```python
from build123d import *

# Parameters (mm, degrees)
SKETCH1_W           = 43
SKETCH1_H           = 68.5
BOSS_EXTRUDE1_DEPTH = 5
SKETCH2_W           = 16
SKETCH2_H           = 68.5
BOSS_EXTRUDE2_DEPTH = 5
CUT_EXTRUDE1_REACH  = 62.855
SKETCH3_R           = 2.35
FILLET1_R           = 1
CHAMFER1_SIZE       = 1


with BuildPart() as part:
    # Sketch1 → Boss-Extrude1 (new body)
    with BuildSketch(Plane(origin=(0, 0, 0), x_dir=(1, 0, 0), z_dir=(0, 1, 0))):
        with Locations((8.893910561, -17.51450999)):
            Rectangle(SKETCH1_W, SKETCH1_H)
    extrude(amount=BOSS_EXTRUDE1_DEPTH)

    # Sketch2 → Boss-Extrude2 (add)
    with BuildSketch(Plane(origin=(0, 5, 0), x_dir=(1, 0, 0), z_dir=(0, 1, 0))):
        with Locations((-15.606089439, -17.51450999)):
            Rectangle(SKETCH2_W, SKETCH2_H)
    boss_extrude2 = extrude(amount=BOSS_EXTRUDE2_DEPTH)

    # Sketch3 → Cut-Extrude1 (cut, up to next)
    with BuildSketch(Plane(origin=(0, 10, 0), x_dir=(1, 0, 0), z_dir=(0, 1, 0)), mode=Mode.PRIVATE) as cut_extrude1_sk1:
        with Locations(Location((-18.106089439, 8.23549001, 0), (0, 0, 270))):
            Circle(SKETCH3_R)
    cut_extrude1_tool1 = extrude(cut_extrude1_sk1.sketch, amount=-CUT_EXTRUDE1_REACH, mode=Mode.PRIVATE) & part.part
    # Sketch3 → Cut-Extrude1 (cut, up to next)
    with BuildSketch(Plane(origin=(0, 10, 0), x_dir=(1, 0, 0), z_dir=(0, 1, 0)), mode=Mode.PRIVATE) as cut_extrude1_sk2:
        with Locations(Location((-18.106089439, -8.931176657, 0), (0, 0, 270))):
            Circle(SKETCH3_R)
    cut_extrude1_tool2 = extrude(cut_extrude1_sk2.sketch, amount=-CUT_EXTRUDE1_REACH, mode=Mode.PRIVATE) & part.part
    # Sketch3 → Cut-Extrude1 (cut, up to next)
    with BuildSketch(Plane(origin=(0, 10, 0), x_dir=(1, 0, 0), z_dir=(0, 1, 0)), mode=Mode.PRIVATE) as cut_extrude1_sk3:
        with Locations(Location((-18.106089439, -26.097843324, 0), (0, 0, 270))):
            Circle(SKETCH3_R)
    cut_extrude1_tool3 = extrude(cut_extrude1_sk3.sketch, amount=-CUT_EXTRUDE1_REACH, mode=Mode.PRIVATE) & part.part
    # Sketch3 → Cut-Extrude1 (cut, up to next)
    with BuildSketch(Plane(origin=(0, 10, 0), x_dir=(1, 0, 0), z_dir=(0, 1, 0)), mode=Mode.PRIVATE) as cut_extrude1_sk4:
        with Locations(Location((-18.106089439, -43.26450999, 0), (0, 0, 270))):
            Circle(SKETCH3_R)
    cut_extrude1_tool4 = extrude(cut_extrude1_sk4.sketch, amount=-CUT_EXTRUDE1_REACH, mode=Mode.PRIVATE) & part.part
    cut_extrude1_1 = cut_extrude1_tool1.solids().sort_by_distance((-18.106089, 10, -8.23549))[0]
    add(cut_extrude1_1, mode=Mode.SUBTRACT)
    cut_extrude1_2 = cut_extrude1_tool2.solids().sort_by_distance((-18.106089, 10, 8.931177))[0]
    add(cut_extrude1_2, mode=Mode.SUBTRACT)
    cut_extrude1_3 = cut_extrude1_tool3.solids().sort_by_distance((-18.106089, 10, 26.097843))[0]
    add(cut_extrude1_3, mode=Mode.SUBTRACT)
    cut_extrude1_4 = cut_extrude1_tool4.solids().sort_by_distance((-18.106089, 10, 43.26451))[0]
    add(cut_extrude1_4, mode=Mode.SUBTRACT)
    cut_extrude1 = cut_extrude1_1 + cut_extrude1_2 + cut_extrude1_3 + cut_extrude1_4  # Cut-Extrude1 as one shape, for the pattern or mirror that repeats it

    # Mirror1: Boss-Extrude2, Cut-Extrude1 across plane
    add(boss_extrude2.mirror(Plane(origin=(8.893910561, 0, 0), x_dir=(0, 0, 1), z_dir=(1, 0, 0))))
    add(cut_extrude1.mirror(Plane(origin=(8.893910561, 0, 0), x_dir=(0, 0, 1), z_dir=(1, 0, 0))), mode=Mode.SUBTRACT)

    # Fillet1
    fillet1_edges = [part.edges().sort_by_distance(p)[0] for p in [
        (30.393910561, 5, 17.51450999),
        (-7.606089439, 5, 17.51450999),
        (-23.606089439, 5, 17.51450999),
        (-7.606089439, 10, 17.51450999),
        (41.393910561, 5, 17.51450999),
        (25.393910561, 10, 17.51450999),
        (-12.606089439, 5, 17.51450999),
        (25.393910561, 5, 17.51450999),
    ]]
    fillet(fillet1_edges, radius=FILLET1_R)

    # Chamfer1
    chamfer1_edges = [part.edges().sort_by_distance(p)[0] for p in [
        (-18.106089439, 5, -10.58549001),
        (-18.106089439, 5, 6.581176657),
        (-18.106089439, 5, 23.747843324),
        (-18.106089439, 5, 40.91450999),
        (35.893910561, 5, -10.58549001),
        (35.893910561, 5, 6.581176657),
        (35.893910561, 5, 23.747843324),
        (35.893910561, 5, 40.91450999),
    ]]
    chamfer(chamfer1_edges, length=CHAMFER1_SIZE)


solid = part.part
```
Here's how the part is built. I have some questions about the finished solid (model axes, mm). A direction names the side the tool comes from. Give positions to 0.01 mm unless a question says otherwise; leave off trailing zeros. Write each loop counter-clockwise with the first axis right and the second up, starting at its lowest first coordinate (ties: lowest second). Pieces come first, ordered by that corner, then holes.
(1) Imagine slicing it at A-A, the plane y = 7. Count the separate pieces of the cut face and the enclosed holes in it, and give its area (3 significant figures).
Output values:
separate pieces: 2
enclosed holes: 8
area: 2,050 mm2
(2) On a 3-axis mill with a long thin cutter (end or side, diameter ignored), from which of +Z, -Z, +X, -X, +Y, -Y can I reach the whole of each face in a straight line? I mean faces 4 (the face through (-18, 5, 17)), 5 (the face through (9, 5, 17)), 6 (the face through (36, 5, 17)). Say none if no direction works.
Output values:
face 4: +Z, -Z, -X, -Y
face 5: +Z, -Z, +Y
face 6: +Z, -Z, +X, -Y
(3) Imagine slicing it at D-D, the plane y = 1. Write out the boundary of the cut face in (x, z).
Output values:
outline: (-12.61, -16.74) - (30.39, -16.74) - (30.39, 51.76) - (-12.61, 51.76) - close
(4) If I drill on L1, parallel to X at y = 8.5, z = -11.5; L2, parallel to Z at x = -19.5, y = 8.25; L3, parallel to X at y = 5.5, z = 8.5, over which ranges is the centre line in solid material (lowest first)?
Output values:
L1: x = -23.61 to -7.61, 25.39 to 41.39
L2: z = -16.74 to -10.13, -6.34 to 7.04, 10.82 to 24.21, 27.99 to 41.37, 45.16 to 51.76
L3: x = -23.47 to -20.92, -15.29 to -7.47, 25.26 to 33.08, 38.71 to 41.26
(5) Imagine slicing it at C-C, the plane x = 8.5. Write out the boundary of the cut face in (y, z), and give its area (4 significant figures).
Output values:
outline: (0, -16.74) - (5, -16.74) - (5, 51.76) - (0, 51.76) - close
area: 342.5 mm2
(6) Thinking about a two-plate mould opening in Z: for faces 1 (the face through (34.306, 8.028, 24.366)), 2 (the face through (9, 4, -16.735)), 3 (the face through (-7.606, 7, 18)), which applies, pulls with the +Z half, pulls with the -Z half, needs draft (parallel to the pull), parting line crosses it, or undercut?
Output values:
face 1: undercut
face 2: pulls with the -Z half
face 3: needs draft
(7) Will these pins go through, and if not, where does the flat tip stop? pin 1 (4 mm diameter, centred on x = 35.89, z = -8.24, fed in from -Y); pin 2 (4.5 mm diameter, centred on y = 2, z = 15.5, fed in from +X); pin 3 (6 mm diameter, centred on x = -18.11, z = 43.26, fed in from -Y); pin 4 (2.5 mm diameter, centred on x = 38, z = 28.5, fed in from -Y).
Output values:
pin 1: passes through
pin 2: stops at x = 30.43
pin 3: stops at y = 5.34
pin 4: stops at y = 5
(8) Imagine slicing it at B-B, the plane z = -3. Write out the boundary of the cut face in (x, y), and give its area (3 significant figures).
Output values:
outline: (-23.61, 6) arc R1 ccw to (-22.61, 5) - (-13.61, 5) arc R1 cw to (-12.61, 4) - (-12.61, 0) - (30.39, 0) - (30.39, 4) arc R1 cw to (31.39, 5) - (40.39, 5) arc R1 ccw to (41.39, 6) - (41.39, 10) - (26.39, 10) arc R1 ccw to (25.39, 9) - (25.39, 6) arc R1 cw to (24.39, 5) - (-6.61, 5) arc R1 cw to (-7.61, 6) - (-7.61, 9) arc R1 ccw to (-8.61, 10) - (-23.61, 10) - close
area: 375 mm2
